```python
from build123d import *

# Parameters (mm, degrees)
SKETCH1_W           = 95
SKETCH1_H           = 82
SKETCH1_R           = 1.1
SKETCH1_R_2         = 1
BOSS_EXTRUDE1_DEPTH = 2
BOSS_EXTRUDE2_DEPTH = 0.2


with BuildPart() as part:
    # Sketch1 → Boss-Extrude1 (new body)
    with BuildSketch(Plane.XY):
        Rectangle(SKETCH1_W, SKETCH1_H)
        with Locations((-43.5, 13.5)):
            Circle(SKETCH1_R, mode=Mode.SUBTRACT)
        with Locations((-43.5, -13.5)):
            Circle(SKETCH1_R, mode=Mode.SUBTRACT)
        with Locations((43.5, 7.5)):
            Circle(SKETCH1_R, mode=Mode.SUBTRACT)
        with Locations((43.5, -7.5)):
            Circle(SKETCH1_R, mode=Mode.SUBTRACT)
        with Locations((-43.5, 7.5)):
            Circle(SKETCH1_R, mode=Mode.SUBTRACT)
        with Locations((-43.5, -7.5)):
            Circle(SKETCH1_R, mode=Mode.SUBTRACT)
        with Locations((43.5, 13.5)):
            Circle(SKETCH1_R, mode=Mode.SUBTRACT)
        with Locations((43.5, -13.5)):
            Circle(SKETCH1_R, mode=Mode.SUBTRACT)
        with Locations((-43.5, -21)):
            Circle(SKETCH1_R_2, mode=Mode.SUBTRACT)
    extrude(amount=BOSS_EXTRUDE1_DEPTH)

    # Sketch2 → Boss-Extrude2 (add)
    with BuildSketch(Plane.XY.offset(2)):
        Polygon((-11, 39.5), (-1, 29.5), (-1, -29.5), (-11, -39.5), (-37.5, -39.5), (-37.5, 39.5), align=None)
        Polygon((1, 39.5), (27.5, 39.5), (37.5, 29.5), (37.5, -29.5), (27.5, -39.5), (1, -39.5), align=None)
    extrude(amount=BOSS_EXTRUDE2_DEPTH)


solid = part.part
```
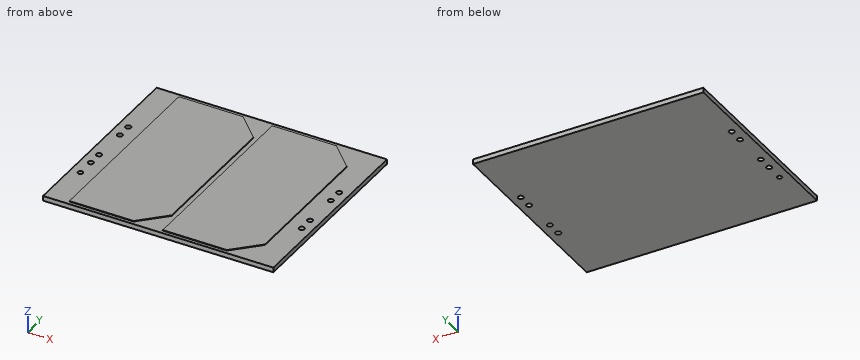
Here's how the part is built. I have some questions about the finished solid (model axes, mm). Coordinates: 2 decimals unless noted, no trailing zeros. Loops run counter-clockwise (first coordinate to the right, second up) from the corner with the lowest first, then second, coordinate; pieces in that order, holes last. Notation, with made-up numbers: (-33, -35.5) - (-16, -35.5) arc R27 cw to (-16, -10.5) - close; hole circle Ø7 at (-11.5, 20.25). An arc over 180 degrees is marked (long way). Return JSON: item names as keys, results as strings. Group by question number.
Item 1: If we section it at C-C on y = 33.5: Write out the boundary of the cut face in (x, z).
Item 2: If we section it at D-D on x = 34: Write out the boundary of the cut face in (y, z), and give its area (3 significant figures).
Item 3: Will this pin go through, and if not, where does the flat tip stop? P1, Ø2.5, axis at x = 43.5, y = 7.5, coming from the +Z side.
Item 4: I need wall thicknesses on line 1 (Y direction, x = 43.5, z = 1.05); line 2 (Y direction, x = -43.5, z = 0.65); line 3 (X direction, y = 1.5, z = 2.15). Which ranges of each line are inside material? Lowest first, please. Write a range as from..to.
Item 5: If we section it at B-B on x = 43.5: Write out the boundary of the cut face in (y, z), and give its area (3 significant figures).
Item 6: If we section it at A-A on y = 7.5: Write out the boundary of the cut face in (x, z).
Calculated:
{
 "1": {"outline": "(-47.5, 0) - (47.5, 0) - (47.5, 2) - (33.5, 2) - (33.5, 2.2) - (1, 2.2) - (1, 2) - (-5, 2) - (-5, 2.2) - (-37.5, 2.2) - (-37.5, 2) - (-47.5, 2) - close"},
 "2": {"outline": "(-41, 0) - (41, 0) - (41, 2) - (33, 2) - (33, 2.2) - (-33, 2.2) - (-33, 2) - (-41, 2) - close", "area": "177 mm^2"},
 "3": {"P1": "stops at z = 2"},
 "4": {"line 1": "y = -41..-14.6, -12.4..-8.6, -6.4..6.4, 8.6..12.4, 14.6..41", "line 2": "y = -41..-22, -20..-14.6, -12.4..-8.6, -6.4..6.4, 8.6..12.4, 14.6..41", "line 3": "x = -37.5..-1, 1..37.5"},
 "5": {"outline": "(-41, 0) - (-14.6, 0) - (-14.6, 2) - (-41, 2) - close; (-12.4, 0) - (-8.6, 0) - (-8.6, 2) - (-12.4, 2) - close; (-6.4, 0) - (6.4, 0) - (6.4, 2) - (-6.4, 2) - close; (8.6, 0) - (12.4, 0) - (12.4, 2) - (8.6, 2) - close; (14.6, 0) - (41, 0) - (41, 2) - (14.6, 2) - close", "area": "146 mm^2"},
 "6": {"outline": "(-47.5, 0) - (-44.6, 0) - (-44.6, 2) - (-47.5, 2) - close; (-42.4, 0) - (42.4, 0) - (42.4, 2) - (37.5, 2) - (37.5, 2.2) - (1, 2.2) - (1, 2) - (-1, 2) - (-1, 2.2) - (-37.5, 2.2) - (-37.5, 2) - (-42.4, 2) - close; (44.6, 0) - (47.5, 0) - (47.5, 2) - (44.6, 2) - close"}
}
